Part model, mm, in its own coordinate system. Face numbers are marked on the shaded views. Give positions to 0.01 mm unless a question says otherwise; leave off trailing zeros. Order: outer loops, then holes, each group sorted by start corner. A loop starts at its lowest first (then second) coordinate and runs counter-clockwise, first axis right, second up. Notation, with made-up numbers: (19, -6.75) - (51, -6.75) arc R23 ccw to (51, 9.25) - close; hole circle Ø3 at (33.25, 64.5). An arc over 180 degrees is marked (long way). Use a Markdown table: item, result. Add a question column.
from build123d import *

# Parameters (mm, degrees)
F0_W     = 77.724
F0_H     = 38.1
F1_DEPTH = 304.8
F3_DEPTH = 609.601
F5_D     = 7.14375


with BuildPart() as f1:
    # F0 (on Right) → F1 (new body, symmetric)
    with BuildSketch(Plane.YZ):
        Rectangle(F0_W, F0_H)
    extrude(amount=F1_DEPTH, both=True)

    # F2 (on face) → F3 (cut, through all)
    with BuildSketch(Plane.YZ.offset(304.8)):
        Polygon((34.925, 19.05), (-34.925, 19.05), (0, 0), align=None)
    extrude(amount=-F3_DEPTH, mode=Mode.SUBTRACT)

    # F5 (through all)
    with Locations(Plane.XZ.offset(38.862)):
        with Locations((-228.6, -9.525), (0, -9.525), (228.6, -9.525), (-279.4, -9.525), (50.8, -9.525)):
            Hole(F5_D / 2)


solid = f1.part
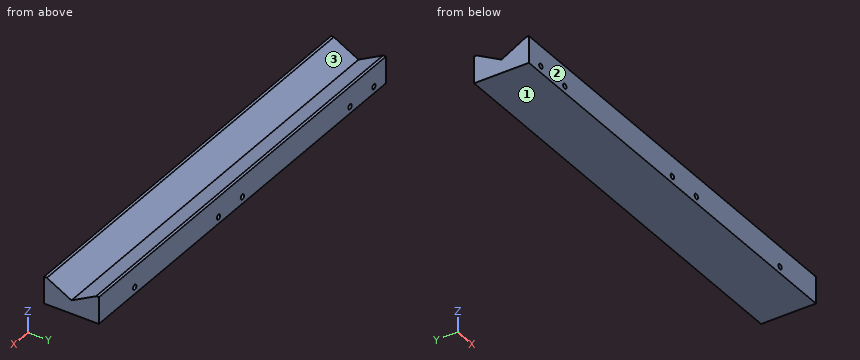
1. Cut at A-A (z = 12). Write the cut outline in (x, y).
2. Drill centre lines: probe 1 along X at (y, z) = (19.5, -9); probe 2 along X at (y, z) = (14, -12); probe 3 along Z at (x, y) = (50, 4). Where is each one in solid material? Low to high. Write a range as [from, to].
3. Mould opens along Y. For the marked faces 1, 2 and 3 say: released by +Y, released by -Y, zero draft, split by the parting line, or undercut.
4. Cut at C-C (x = 178). Write the cut outline in (y, z) (3 decimals), plus the area to 3 significant figures.
5. Cut at B-B (y = 13.5). Write the cut outline in (x, z) (3 decimals), plus the area to 3 significant figures.
6. Pin check, flat tips, straight feed: P1, Ø6, axis at x = 112.5, y = 16, coming from the +Z side; P2, Ø5.5, axis at x = 228.6, z = -9.525, coming from the -Y side; P3, Ø5, axis at x = -16, y = 25, coming from the +Z side; P4, Ø10, axis at x = -86.5, y = 20.5, coming from the +Z side. Stop position of each tip, or through.
Responses:
| question | item | result |
|---|---|---|
| 1 | outline | (-304.8, -38.86) - (304.8, -38.86) - (304.8, -22) - (-304.8, -22) - close; (-304.8, 22) - (304.8, 22) - (304.8, 38.86) - (-304.8, 38.86) - close |
| 2 | probe 1 | x = [-304.8, -282.93], [-275.87, -232.13], [-225.07, -3.53], [3.53, 47.27], [54.33, 225.07], [232.13, 304.8] |
| 2 | probe 2 | x = [-304.8, -281.98], [-276.82, -231.18], [-226.02, -2.58], [2.58, 48.22], [53.38, 226.02], [231.18, 304.8] |
| 2 | probe 3 | z = [-19.05, -13.01], [-6.04, 2.18] |
| 3 | face 1 | zero draft |
| 3 | face 2 | released by -Y |
| 3 | face 3 | undercut |
| 4 | outline | (-38.862, -19.05) - (38.862, -19.05) - (38.862, 19.05) - (34.925, 19.05) - (0, 0) - (-34.925, 19.05) - (-38.862, 19.05) - close |
| 4 | area | 2,300 mm² |
| 5 | outline | (-304.8, -19.05) - (304.8, -19.05) - (304.8, 7.364) - (-304.8, 7.364) - close; hole circle Ø7.144 at (-279.4, -9.525); hole circle Ø7.144 at (-228.6, -9.525); hole circle Ø7.144 at (0, -9.525); hole circle Ø7.144 at (50.8, -9.525); hole circle Ø7.144 at (228.6, -9.525) |
| 5 | area | 15,900 mm² |
| 6 | P1 | stops at z = 10.36 |
| 6 | P2 | passes through |
| 6 | P3 | stops at z = 15 |
| 6 | P4 | stops at z = 13.91 |
